Geometry: final body of the model. Coordinates: model frame, mm. Face numbers are marked on the shaded views. A direction names the side the tool comes from. Round coordinates to 2 decimals unless told otherwise and drop trailing zeros. Write each loop counter-clockwise with the first axis right and the second up, starting at its lowest first coordinate (ties: lowest second). Pieces come first, ordered by that corner, then holes. Notation, with made-up numbers: M 64.5,59 L 101.5,59 A13 ccw 101.5,80 Z; hole C 10,75 d8. An arc over 180 degrees is marked long. Answer as CSV lines item,"result". Start each with the question number.
Q1. Reachability of the marked faces 1, 2 and 3 from +Z, -Z, +X, -X, +Y, -Y: full face, straight path, thin tool, end or side. Return the list, or none.
Q2. Section query B-B on y = -50. Output: boundary loops of the cut face in (x, z).
Q3. First-contact query: pin 1 (1.4 mm diameter, centred on y = -57, z = 5.5, fed in from -X); pin 2 (2.5 mm diameter, centred on y = -55, z = 5, fed in from +X); pin 3 (2.5 mm diameter, centred on y = -48, z = 3.5, fed in from +X). Flat tips, straight axial feed; report the tip coordinate or a pass-through.
Q4. Section query D-D on z = 6.5. Output: boundary loops of the cut face in (x, y).
Q5. Section query C-C on x = 12. Output: boundary loops of the cut face in (y, z).
Q6. Ray query, probe 1 along X at (y, z) = (-33.5, 1); probe 2 along Z at (x, y) = (-2, -49.25); probe 3 along X at (y, z) = (-49.25, 2). Return the intervals inside material, ascending.
Q7. Section query A-A on z = 2.5. Output: boundary loops of the cut face in (x, y).
```python
from build123d import *

# Parameters (mm, degrees)
SKETCH_1_R      = 1
EXTRUDE_1_DEPTH = 1.5
SKETCH_2_W      = 23
SKETCH_2_H      = 12.5
EXTRUDE_2_DEPTH = 3
SKETCH_3_W      = 6
SKETCH_3_H      = 4.6
EXTRUDE_3_DEPTH = 6


with BuildPart() as part:
    # 草圖1 → 填料-伸長1 (new body)
    with BuildSketch(Plane.XY):
        with BuildLine():
            Line((-33.501650513, -58.056539749), (32.498349487, -58.056539749))
            ThreePointArc((32.498349487, -58.056539749), (33.205456268, -57.76364653), (33.498349487, -57.056539749))
            Line((33.498349487, -57.056539749), (33.498349487, -33.056539749))
            ThreePointArc((33.498349487, -33.056539749), (33.205456268, -32.349432967), (32.498349487, -32.056539749))
            Line((32.498349487, -32.056539749), (-33.501650513, -32.056539749))
            ThreePointArc((-33.501650513, -32.056539749), (-34.208757294, -32.349432967), (-34.501650513, -33.056539749))
            Line((-34.501650513, -33.056539749), (-34.501650513, -57.056539749))
            ThreePointArc((-34.501650513, -57.056539749), (-34.208757294, -57.76364653), (-33.501650513, -58.056539749))
        make_face()
        with Locations((-32.501650513, -34.056539749)):
            Circle(SKETCH_1_R, mode=Mode.SUBTRACT)
        with Locations((-32.501650513, -56.056539749)):
            Circle(SKETCH_1_R, mode=Mode.SUBTRACT)
        with Locations((31.498349487, -56.056539749)):
            Circle(SKETCH_1_R, mode=Mode.SUBTRACT)
        with Locations((31.498349487, -34.056539749)):
            Circle(SKETCH_1_R, mode=Mode.SUBTRACT)
    extrude(amount=EXTRUDE_1_DEPTH)

    # 草圖2 → 填料-伸長2 (add)
    with BuildSketch(Plane.XY.offset(1.5)):
        with Locations((17.998349487, -45.056539749)):
            Rectangle(SKETCH_2_W, SKETCH_2_H)
    extrude(amount=EXTRUDE_2_DEPTH)

    # 草圖3 → 填料-伸長3 (add)
    with BuildSketch(Plane.XY.offset(1.5)):
        with Locations((-22.901650513, -55.756539749)):
            Rectangle(SKETCH_3_W, SKETCH_3_H)
    extrude(amount=EXTRUDE_3_DEPTH)


solid = part.part
```
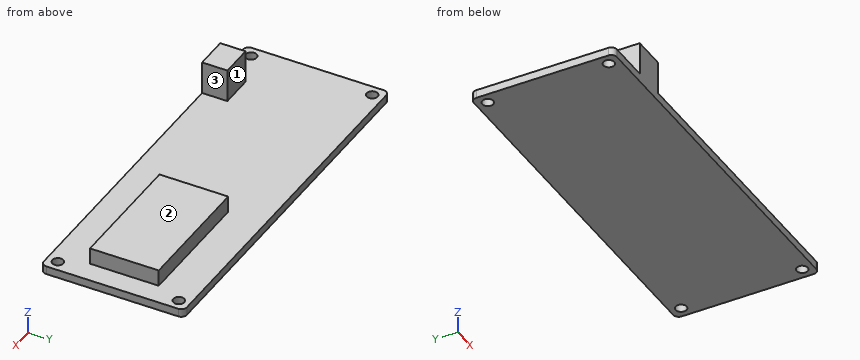
Entries:
1,face 1,"+Z, +X, -X, +Y"
1,face 2,"+Z, +X, -X, +Y, -Y"
1,face 3,"+Z, +X, +Y, -Y"
2,outline,"M -34.5,0 L 33.5,0 L 33.5,1.5 L 29.5,1.5 L 29.5,4.5 L 6.5,4.5 L 6.5,1.5 L -34.5,1.5 Z"
3,pin 1,"stops at x = -25.9"
3,pin 2,"stops at x = -19.9"
3,pin 3,"stops at x = 29.5"
4,outline,"M -25.9,-58.06 L -19.9,-58.06 L -19.9,-53.46 L -25.9,-53.46 Z"
5,outline,"M -58.06,0 L -32.06,0 L -32.06,1.5 L -38.81,1.5 L -38.81,4.5 L -51.31,4.5 L -51.31,1.5 L -58.06,1.5 Z"
6,probe 1,"x = -34.5 to -33.33, -31.67 to 30.67, 32.33 to 33.5"
6,probe 2,"z = 0 to 1.5"
6,probe 3,"x = 6.5 to 29.5"
7,outline,"M -25.9,-58.06 L -19.9,-58.06 L -19.9,-53.46 L -25.9,-53.46 Z; M 6.5,-51.31 L 29.5,-51.31 L 29.5,-38.81 L 6.5,-38.81 Z"
